from build123d import *

# Parameters (mm, degrees)
F0_R     = 4
F1_DEPTH = 3.5
F0_R_2   = 11
F2_DEPTH = 1
F4_DEPTH = 0.5


# Not quite as in the source:
# - a fillet or chamfer that OpenCascade refuses, or shapes differently, is made with other operations: its cross-section is extruded or revolved along the edge and cut away or added


with BuildPart() as f1:
    # F0 (on Top) → F1 (new body)
    with BuildSketch(Plane.XY):
        Circle(F0_R)
    extrude(amount=F1_DEPTH)

    # F0 (on Top) → F2 (join)
    with BuildSketch(Plane.XY):
        Circle(F0_R_2)
        Circle(F0_R, mode=Mode.SUBTRACT)
    extrude(amount=F2_DEPTH)

    # F3 (on face) → F4 (cut)
    with BuildSketch(Plane.XY):
        with BuildLine():
            Line((-0.6011938094, -3.9545626817), (-0.6011938094, -7.9646864906))
            ThreePointArc((-0.6011938094, -7.9646864906), (0, -8.523200555), (0.6011938094, -7.9646864906))
            Line((0.6011938094, -7.9646864906), (0.6011938094, -3.9545626817))
            ThreePointArc((0.6011938094, -3.9545626817), (0, -4), (-0.6011938094, -3.9545626817))
        make_face()
        with BuildLine():
            Line((-0.6011938094, 0), (-0.6011938094, -3.9545626817))
            ThreePointArc((-0.6011938094, -3.9545626817), (0, -4), (0.6011938094, -3.9545626817))
            Line((0.6011938094, -3.9545626817), (0.6011938094, 0))
            ThreePointArc((0.6011938094, 0), (0, 0.6491973737), (-0.6011938094, 0))
        make_face()
        with BuildLine():
            ThreePointArc((-1.7606344773, -6.5513337031), (0, 6.8746740692), (1.7606344773, -6.5513337031))
            ThreePointArc((1.7606344773, -6.5513337031), (1.5154543616, -7.2599851451), (2.1851049368, -7.5974288625))
            ThreePointArc((2.1851049368, -7.5974288625), (2.2008228493, -7.5929180655), (2.21653145, -7.5883749472))
            ThreePointArc((2.21653145, -7.5883749472), (0, 7.9960832706), (-2.21653145, -7.5883749472))
            ThreePointArc((-2.21653145, -7.5883749472), (-2.2008228493, -7.5929180655), (-2.1851049368, -7.5974288625))
            ThreePointArc((-2.1851049368, -7.5974288625), (-1.5154543616, -7.2599851451), (-1.7606344773, -6.5513337031))
        make_face()
    extrude(amount=F4_DEPTH, mode=Mode.SUBTRACT)

    # F5: fillet of radius 5.08 on 1 edges, made by hand

    # F5_s1 → F5_t2 (revolve, cut)
    with BuildSketch(Plane.XZ):
        with BuildLine():
            ThreePointArc((11, 1), (9.567188555, 0.2564743185), (7.9734508099, 0))
            Line((7.9734508099, 0), (11, 0))
            Line((11, 0), (11, 1))
        make_face()
    revolve(axis=Axis((0, 0, 0), (0, 0, 1)), mode=Mode.SUBTRACT)


solid = f1.part
Could you check a few things on this model? Use its own coordinates, in mm. A direction names the side the tool comes from. Round coordinates to 2 decimals unless told otherwise and drop trailing zeros. Write each loop counter-clockwise with the first axis right and the second up, starting at its lowest first coordinate (ties: lowest second). Pieces come first, ordered by that corner, then holes. Notation, with made-up numbers: (60.25, 66) - (105.25, 66) arc R23 cw to (105.25, 82) - close; hole circle Ø8 at (-33, 27). An arc over 180 degrees is marked (long way). Put each result on its own line as item: value. Start each with the question number.
(1) I want a section at A-A, the plane x = 0. Please give me the cut outline in (y, z).
(2) For faces 4 (the cylindrical face through (0.32, 7.99, 0.25)), 5 (the flat face through (0, 1, 0)), which set-ups out of +Z, -Z, +X, -X, +Y, -Y let a thin tool reach every point of the face, with its end or its side?
(3) Thinking about a two-plate mould opening in Y: for faces 1 (the flat face through (0, -5, 1)), 2 (the cylindrical face through (-0.867, -3.905, 2.232)), 3 (the flat face through (0, -4, 0.5)), which applies, released by +Y, released by -Y, zero draft, split by the parting line, or undercut?
(4) I want a section at B-B, the plane z = 3. Please give me the cut outline in (x, y).
(5) I need wall thicknesses on probe 1 along Z at (x, y) = (4.75, 1.5); probe 2 along Z at (x, y) = (5.25, -5.25); probe 3 along X at (y, z) = (-3.25, 2.9). Which ranges of each line are inside material? Lowest first, please.
(6) Will these pins go through, and if not, where does the flat tip stop? pin 1 (1 mm diameter, centred on y = -4, z = 2.5, fed in from +X); pin 2 (1 mm diameter, centred on y = 5, z = 1, fed in from +X).
Here are the results:
1. outline: (-11, 1) arc R5.08 ccw to (-8.52, 0.03) - (-8.52, 0.5) - (0.65, 0.5) - (0.65, 0) - (6.87, 0) - (6.87, 0.5) - (8, 0.5) - (8, 0) arc R5.08 ccw to (11, 1) - (4, 1) - (4, 3.5) - (-4, 3.5) - (-4, 1) - close
2. face 4: -Z
2. face 5: -Z, +X, -X, +Y, -Y
3. face 1: zero draft
3. face 2: split by the parting line
3. face 3: undercut
4. outline: circle Ø8 at (0, 0)
5. probe 1: z = 0 to 1
5. probe 2: z = 0.5 to 1
5. probe 3: x = -2.33 to 2.33
6. pin 1: stops at x = 1.94
6. pin 2: stops at x = 10.04
